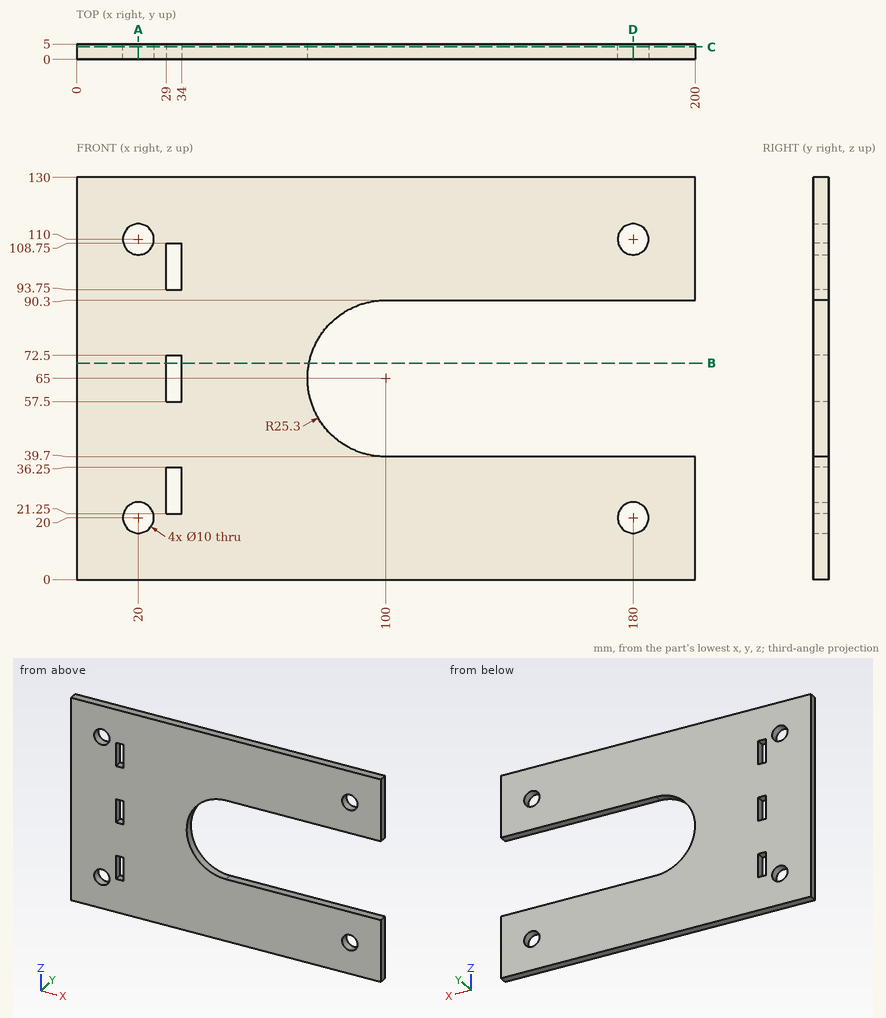
Design review of the part shown in the three views and the two pictorial views. Dimensions are in mm from the part's minimum x, y and z. Give positions to 0.01 mm unless a question says otherwise; leave off trailing zeros. Loops run counter-clockwise (first coordinate to the right, second up) from the corner with the lowest first, then second, coordinate; pieces in that order, holes last. Notation, with made-up numbers: M -1,89.25 L 6,89.25 A13 ccw 6,98.25 Z; hole C 7.5,1.5 d11. An arc over 180 degrees is marked long. Answer as a JSON object with one key per item and string values. Group by question number.
Q1. Add section B-B on z = 70. Give the boundary of the cut face in (x, y), and give its area (3 significant figures).
Q2. Insertion check: P1, Ø6, axis at x = 20, z = 110, coming from the +Y side; P2, Ø1.5, axis at y = 2.5, z = 67.5, coming from the +X side. Each pin has a flat end and moves straight along its axis. Give the tip position at first contact, or say it passes through.
Q3. Add section D-D on x = 180. Give the boundary of the cut face in (y, z).
Q4. For probe 1 along Z at (x, y) = (180, 2.4); probe 2 along Z at (x, y) = (20, 3.05); probe 3 along Z at (x, y) = (166, 0.9), list the stretches that pass through material, from the lowest coordinate up. Write a range as [from, to].
Q5. Add section A-A on x = 20. Give the boundary of the cut face in (y, z), and give its area (3 significant figures).
Q6. Add section C-C on y = 4.05. Give the boundary of the cut face in (x, z), and give its area (3 significant figures).
Checked values:
{
 "1": {"outline": "M 0,0 L 29,0 L 29,5 L 0,5 Z; M 34,0 L 75.2,0 L 75.2,5 L 34,5 Z", "area": "351 mm²"},
 "2": {"P1": "through", "P2": "x = 74.91"},
 "3": {"outline": "M 0,0 L 5,0 L 5,15 L 0,15 Z; M 0,25 L 5,25 L 5,39.7 L 0,39.7 Z; M 0,90.3 L 5,90.3 L 5,105 L 0,105 Z; M 0,115 L 5,115 L 5,130 L 0,130 Z"},
 "4": {"probe 1": "[0, 15], [25, 39.7], [90.3, 105], [115, 130]", "probe 2": "[0, 15], [25, 105], [115, 130]", "probe 3": "[0, 39.7], [90.3, 130]"},
 "5": {"outline": "M 0,0 L 5,0 L 5,15 L 0,15 Z; M 0,25 L 5,25 L 5,105 L 0,105 Z; M 0,115 L 5,115 L 5,130 L 0,130 Z", "area": "550 mm²"},
 "6": {"outline": "M 0,0 L 200,0 L 200,39.7 L 100,39.7 A25.3 cw 100,90.3 L 200,90.3 L 200,130 L 0,130 Z; hole C 20,20 d10; hole C 20,110 d10; hole M 29,21.25 L 34,21.25 L 34,36.25 L 29,36.25 Z; hole M 29,57.5 L 34,57.5 L 34,72.5 L 29,72.5 Z; hole M 29,93.75 L 34,93.75 L 34,108.75 L 29,108.75 Z; hole C 180,20 d10; hole C 180,110 d10", "area": "19,400 mm²"}
}
